Can you work these out from the drawing? Everything is in mm from the part's minimum corner. Give positions to 0.01 mm unless a question says otherwise; leave off trailing zeros. Loops run counter-clockwise (first coordinate to the right, second up) from the corner with the lowest first, then second, coordinate; pieces in that order, holes last. Notation, with made-up numbers: M -36,13.5 L 17,13.5 A26 ccw 17,38.5 Z; hole C 74.5,63 d7. An arc over 180 degrees is marked long. Use CSV: the item, a comma, the result in double quotes.
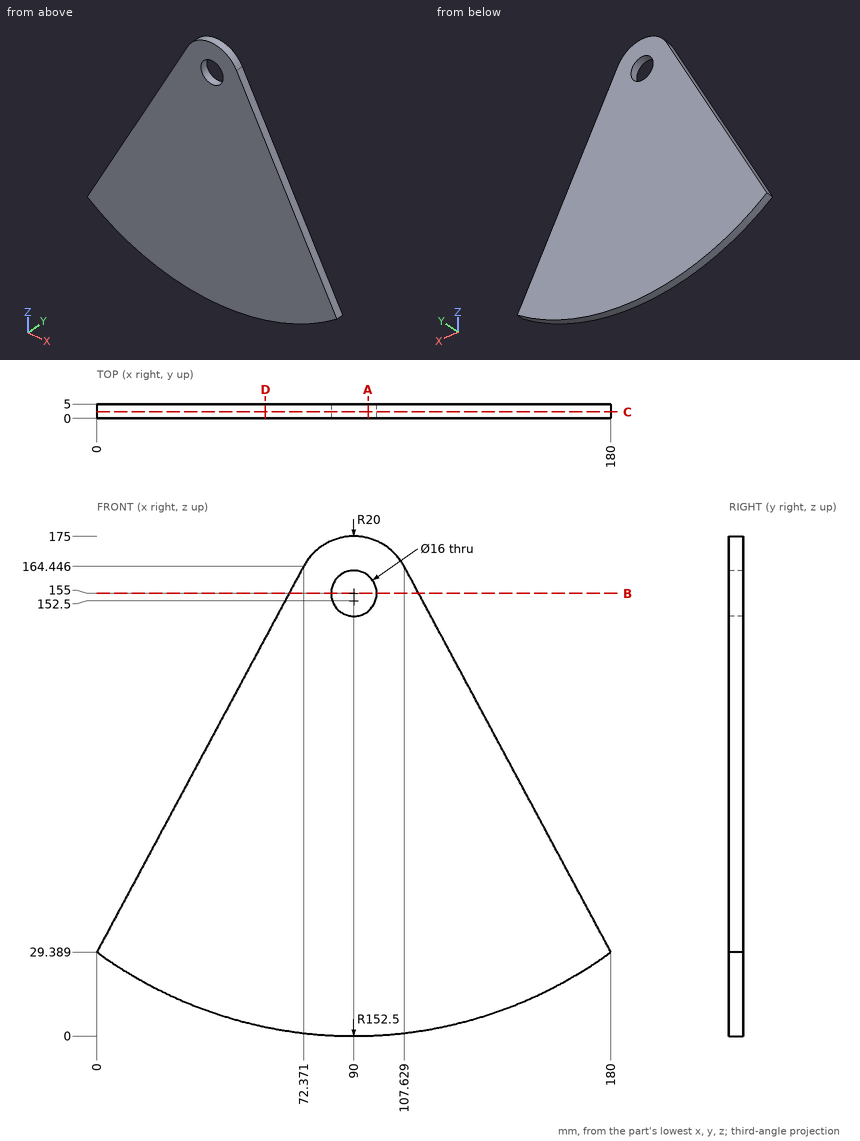
Q1. I want a section at C-C, the plane y = 2.25. Please give me the cut outline in (x, z).
Model answer:
outline,"M 0,29.39 A152.5 ccw 180,29.39 L 107.63,164.45 A20 ccw 72.37,164.45 Z; hole C 90,155 d16"
Q2. Please list where these lines run through material, in increasing order: L1, parallel to X at y = 3.3, z = 37; L2, parallel to Z at x = 131, y = 1.95 (1 decimal); L3, parallel to X at y = 4.85, z = 97. Write a range as from..to.
Model answer:
L1,"4.08..175.92"
L2,"5.6..120.8"
L3,"36.23..143.77"
Q3. I want a section at A-A, the plane x = 95. Please give me the cut outline in (y, z) (1 decimal).
Model answer:
outline,"M 0,0.1 L 5,0.1 L 5,148.8 L 0,148.8 Z; M 0,161.2 L 5,161.2 L 5,174.4 L 0,174.4 Z"
Q4. I want a section at D-D, the plane x = 59. Please give me the cut outline in (y, z).
Model answer:
outline,"M 0,3.18 L 5,3.18 L 5,139.49 L 0,139.49 Z"
Q5. I want a section at B-B, the plane z = 155. Please give me the cut outline in (x, y).
Model answer:
outline,"M 67.31,0 L 82,0 L 82,5 L 67.31,5 Z; M 98,0 L 112.69,0 L 112.69,5 L 98,5 Z"
